from build123d import *

# Parameters (mm, degrees)
SKETCH_1_W          = 15
SKETCH_1_H          = 15
EXTRUDE_1_DEPTH     = 95
SKETCH_2_R          = 1.7
CUT_EXTRUDE_1_DEPTH = 98.33961167
SKETCH_3_R          = 1.7
CUT_EXTRUDE_2_DEPTH = 98.33961167


with BuildPart() as part:
    # 草图1 → 凸台-拉伸1 (new body)
    with BuildSketch(Plane(origin=(0, 0, 0), x_dir=(1, 0, 0), z_dir=(0, 1, 0))):
        with Locations((7.5, 7.5)):
            Rectangle(SKETCH_1_W, SKETCH_1_H)
    extrude(amount=EXTRUDE_1_DEPTH)

    # 草图2 → 切除-拉伸1 (cut, through all)
    with BuildSketch(Plane.XY):
        with Locations((7.5, 10)):
            Circle(SKETCH_2_R)
        with Locations((7.5, 30)):
            Circle(SKETCH_2_R)
    extrude(amount=-CUT_EXTRUDE_1_DEPTH, mode=Mode.SUBTRACT)

    # 草图3 → 切除-拉伸2 (cut, through all)
    with BuildSketch(Plane(origin=(15, 0, 0), x_dir=(0, 0, -1), z_dir=(1, 0, 0))):
        with Locations((7.5, 85)):
            Circle(SKETCH_3_R)
        with Locations((7.5, 65)):
            Circle(SKETCH_3_R)
    extrude(amount=-CUT_EXTRUDE_2_DEPTH, mode=Mode.SUBTRACT)


solid = part.part
Work out the finished part from the listing and answer in its coordinate system (mm). Give positions to 0.01 mm unless a question says otherwise; leave off trailing zeros. Write each loop counter-clockwise with the first axis right and the second up, starting at its lowest first coordinate (ties: lowest second). Pieces come first, ordered by that corner, then holes. Notation, with made-up numbers: (-30, 3) - (-15, 3) arc R19 cw to (-15, 28) - close; hole circle Ø10 at (51.5, 26.25). An arc over 180 degrees is marked (long way). One line per item, written item: value. Start each with the question number.
1. For a pull along Z with two mould halves and no side action, classify faces 1 (the cylindrical face through (7.6, 66.15, -6.25)), 2 (the flat face through (7, 95, -8)), 3 (the flat face through (7, 47, -15)) as +Z half, -Z half, draft (parallel to the pull), parting line (faces both ways), or undercut.
2. Find section B-B (y = 30). Write down the section's boundary in (x, z).
3. Find section A-A (x = 7.5). Write down the section's boundary in (y, z), then the cut area to 3 significant figures.
4. Consider probe 1 along Y at (x, z) = (3.25, -8); probe 2 along Y at (x, z) = (7, -10.5); probe 3 along Z at (x, y) = (4.25, 85). Determine where each line is inside the solid, lowest interval first.
5. Find section C-C (z = -7.5). Write down the section's boundary in (x, y).
Geometry results:
1. face 1: undercut
1. face 2: draft
1. face 3: -Z half
2. outline: (0, -15) - (5.8, -15) - (5.8, 0) - (0, 0) - close; (9.2, -15) - (15, -15) - (15, 0) - (9.2, 0) - close
3. outline: (0, -15) - (8.3, -15) - (8.3, 0) - (0, 0) - close; (11.7, -15) - (28.3, -15) - (28.3, 0) - (11.7, 0) - close; (31.7, -15) - (95, -15) - (95, 0) - (31.7, 0) - close; hole circle Ø3.4 at (65, -7.5); hole circle Ø3.4 at (85, -7.5)
3. area: 1,300 mm2
4. probe 1: 0 to 63.38, 66.62 to 83.38, 86.62 to 95
4. probe 2: 0 to 8.38, 11.62 to 28.38, 31.62 to 95
4. probe 3: -15 to -9.2, -5.8 to 0
5. outline: (0, 0) - (15, 0) - (15, 63.3) - (0, 63.3) - close; (0, 66.7) - (15, 66.7) - (15, 83.3) - (0, 83.3) - close; (0, 86.7) - (15, 86.7) - (15, 95) - (0, 95) - close; hole circle Ø3.4 at (7.5, 10); hole circle Ø3.4 at (7.5, 30)
